The drawing under review shows one solid part. Ordinate dimensions are in mm from its lowest x, y, z. A direction names the side the tool comes from. Round coordinates to 2 decimals unless told otherwise and drop trailing zeros. Order: outer loops, then holes, each group sorted by start corner. A loop starts at its lowest first (then second) coordinate and runs counter-clockwise, first axis right, second up. Notation, with made-up numbers: (42, 62.5) -> (70, 62.5) arc R11 ccw to (70, 66.5) -> close; hole circle Ø6 at (19.25, -19). An arc over 180 degrees is marked (long way). Use a Markdown table: item, result. Add a question column.
1) Consider section A-A (z = 24). State the section outline as (x, y) points.
2) Clearance check with flat-ended pins moving along their axes: P1, Ø1, axis at y = 3.5, z = 10.5, coming from the +X side; P2, Ø3, axis at x = 15, y = 2, coming from the -Z side. State where each tip first meets the part, or that it passes through.
3) Consider section B-B (x = 4.25). State the section outline as (y, z) points.
4) Machinability: for the marked faces 1, 2 and 3, which of the approach directions +Z, -Z, +X, -X, +Y, -Y give a long, thin tool a straight path to every point of the face, cutting with its end or side? Answer none if there is none.
5) Wall thickness on line 1 along Z through (x, y) = (14.75, 0.6); line 2 along Z through (x, y) = (9.75, 4.8); line 3 along X through (y, z) = (5.15, 35): over which ranges is each line inside the solid? List them lowest first. Write a range as [from, to].
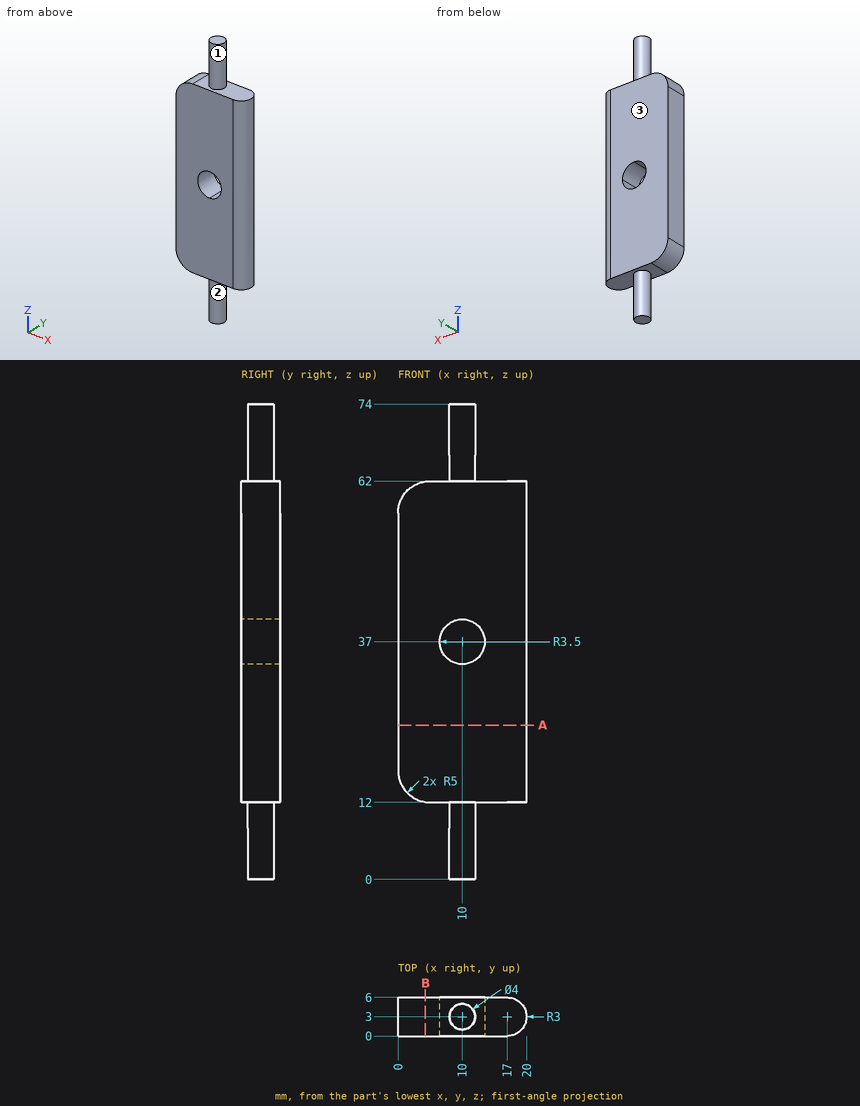
Results list:
| question | item | result |
|---|---|---|
| 1 | outline | (0, 0) -> (17, 0) arc R3 ccw to (17, 6) -> (0, 6) -> close |
| 2 | P1 | x = 12 |
| 2 | P2 | z = 12 |
| 3 | outline | (0, 12.06) -> (6, 12.06) -> (6, 61.94) -> (0, 61.94) -> close |
| 4 | face 1 | +Z |
| 4 | face 2 | -Z |
| 4 | face 3 | +Z, -Z, +X, -X, +Y |
| 5 | line 1 | [12, 62] |
| 5 | line 2 | [0, 33.51], [40.49, 74] |
| 5 | line 3 | [0, 7.13], [12.87, 19.09] |
